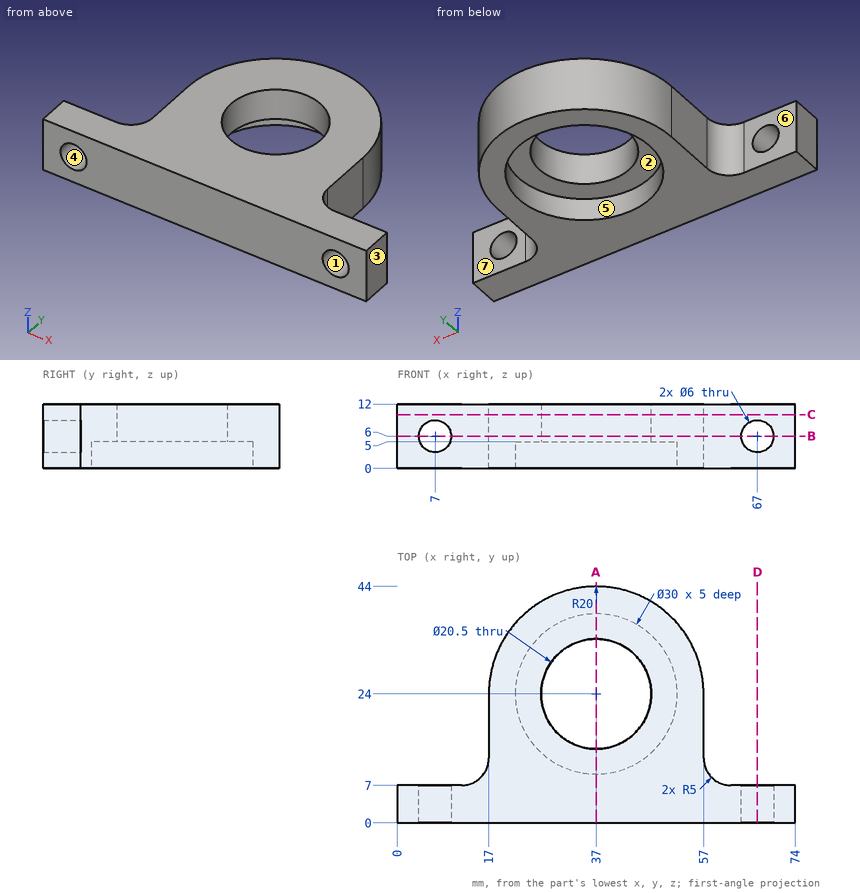
Source: three-view drawing plus pictorial views. Frame: mm from the lowest corner of the part. A direction names the side the tool comes from. Coordinates: 2 decimals unless noted, no trailing zeros. Order: outer loops, then holes, each group sorted by start corner. A loop starts at its lowest first (then second) coordinate and runs counter-clockwise, first axis right, second up. Notation, with made-up numbers: M 42.25,41 L 98.25,41 A22 cw 98.25,71 Z; hole C 3,-9 d3. An arc over 180 degrees is marked long. One line per question, with ' | ' between items. Start each with the question number.
Item 1: Pin query (flat end, axial travel): pin 1 Ø5 at (x, z) = (7, 6) entering from -Y; pin 2 Ø2 at (x, z) = (56.5, 10) entering from +Y; pin 3 Ø6 at (y, z) = (20.5, 7) entering from -X; pin 4 Ø1.5 at (y, z) = (9.5, 7.5) entering from +X. Return the tip coordinate at first contact, or that it passes through.
Item 2: Cut plane C-C, the plane z = 10. Return the cut outline in (x, y), then the cut area to 3 significant figures.
Item 3: Cut plane A-A, the plane x = 37. Return the cut outline in (y, z), then the cut area to 4 significant figures.
Item 4: Cut plane D-D, the plane x = 67. Return the cut outline in (y, z).
Item 5: Draft query along Z for the marked faces 1, 2, 3 and 4. Return one class per face: released by +Z, released by -Z, zero draft, split by the parting line, or undercut.
Item 6: Set-up query: the marked faces 5, 6 and 7. Return all of +Z, -Z, +X, -X, +Y, -Y with unobstructed straight access to the full face (end or side cutting, diameter ignored); none if empty.
Item 7: Ray query, probe 1 along X at (y, z) = (4.75, 6); probe 2 along Y at (x, z) = (37, 2.1); probe 3 along X at (y, z) = (24, 7.5). Return the intervals inside material, ascending. Write a range as [from, to].
Item 8: Cut plane B-B, the plane z = 6. Return the cut outline in (x, y), then the cut area to 3 significant figures.
A:
1) pin 1: passes through | pin 2: stops at y = 31.6 | pin 3: stops at x = 17 | pin 4: stops at x = 58.2
2) outline: M 0,0 L 74,0 L 74,7 L 62,7 A5 cw 57,12 L 57,24 A20 ccw 17,24 L 17,12 A5 cw 12,7 L 0,7 Z; hole C 37,24 d20.5 | area: 1,510 mm2
3) outline: M 0,0 L 9,0 L 9,5 L 13.75,5 L 13.75,12 L 0,12 Z; M 34.25,5 L 39,5 L 39,0 L 44,0 L 44,12 L 34.25,12 Z | area: 234.5 mm2
4) outline: M 0,0 L 7,0 L 7,3 L 0,3 Z; M 0,9 L 7,9 L 7,12 L 0,12 Z
5) face 1: undercut | face 2: released by -Z | face 3: zero draft | face 4: undercut
6) face 5: -Z | face 6: +Z, -Z, -X, +Y | face 7: +Z, -Z, +X, +Y
7) probe 1: x = [0, 4], [10, 64], [70, 74] | probe 2: y = [0, 9], [39, 44] | probe 3: x = [17, 26.75], [47.25, 57]
8) outline: M 0,0 L 4,0 L 4,7 L 0,7 Z; M 10,0 L 64,0 L 64,7 L 62,7 A5 cw 57,12 L 57,24 A20 ccw 17,24 L 17,12 A5 cw 12,7 L 10,7 Z; M 70,0 L 74,0 L 74,7 L 70,7 Z; hole C 37,24 d20.5 | area: 1,420 mm2
